The figure shows three views and two pictorial views of one solid part (mm, origin at its lowest corner). Answer the questions. Give positions to 0.01 mm unless a question says otherwise; leave off trailing zeros. Write each loop counter-clockwise with the first axis right and the second up, starting at its lowest first coordinate (ties: lowest second). Pieces come first, ordered by that corner, then holes. Notation, with made-up numbers: (-36.5, 41) -> (4.5, 41) arc R23 ccw to (4.5, 51) -> close; hole circle Ø2 at (65.25, 74). An arc over 180 degrees is marked (long way). Use a Markdown table: item, result.
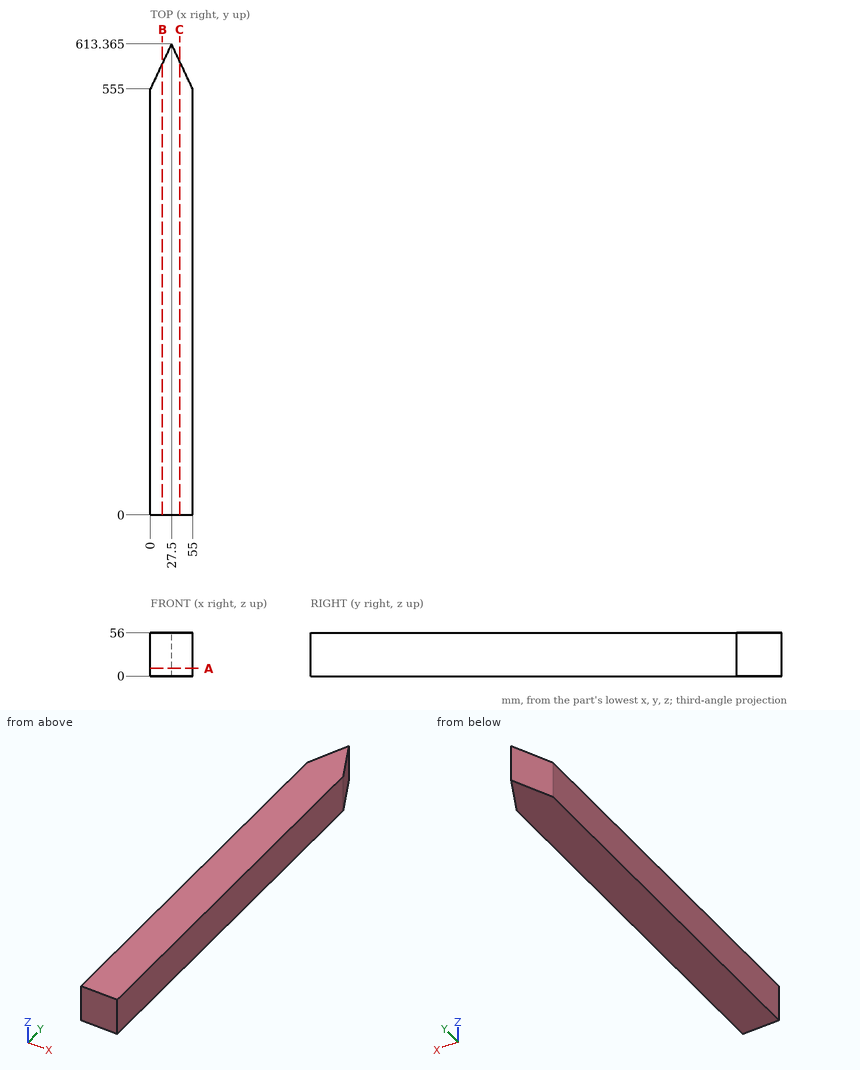
Item 1: Straight lines are drawn through the part: line 1 along Y through (x, z) = (8.5, 20); line 2 along Y through (x, z) = (38, 30); line 3 along X through (y, z) = (585.5, 3). For each, find the intervals that lie inside material, in ascending order. Write a range as [from, to].
Return value:
| item | result |
|---|---|
| line 1 | [0, 573.04] |
| line 2 | [0, 591.08] |
| line 3 | [14.37, 40.63] |
Item 2: A cutting plane is placed at A-A (z = 10). Give the vertices of the cut face in (x, y) (1 decimal), then the cut area to 3 significant figures.
Return value:
| item | result |
|---|---|
| outline | (0, 0) -> (55, 0) -> (55, 555) -> (27.5, 613.4) -> (0, 555) -> close |
| area | 32,100 mm^2 |
Item 3: A cutting plane is placed at C-C (x = 38). Give the vertices of the cut face in (y, z), then the cut area to 3 significant figures.
Return value:
| item | result |
|---|---|
| outline | (0, 0) -> (591.08, 0) -> (591.08, 56) -> (0, 56) -> close |
| area | 33,100 mm^2 |
Item 4: A cutting plane is placed at B-B (x = 15.5). Give the vertices of the cut face in (y, z).
Return value:
| item | result |
|---|---|
| outline | (0, 0) -> (587.9, 0) -> (587.9, 56) -> (0, 56) -> close |
Item 5: Each of these flat-tipped pins is pushed along its axis until it touches: P1, Ø6, axis at x = 47.5, z = 33, coming from the +Y side (1 decimal); P2, Ø5, axis at x = 10, z = 19, coming from the +Y side. Where does it stop, or does it pass through?
Return value:
| item | result |
|---|---|
| P1 | y = 577.3 |
| P2 | y = 581.53 |
